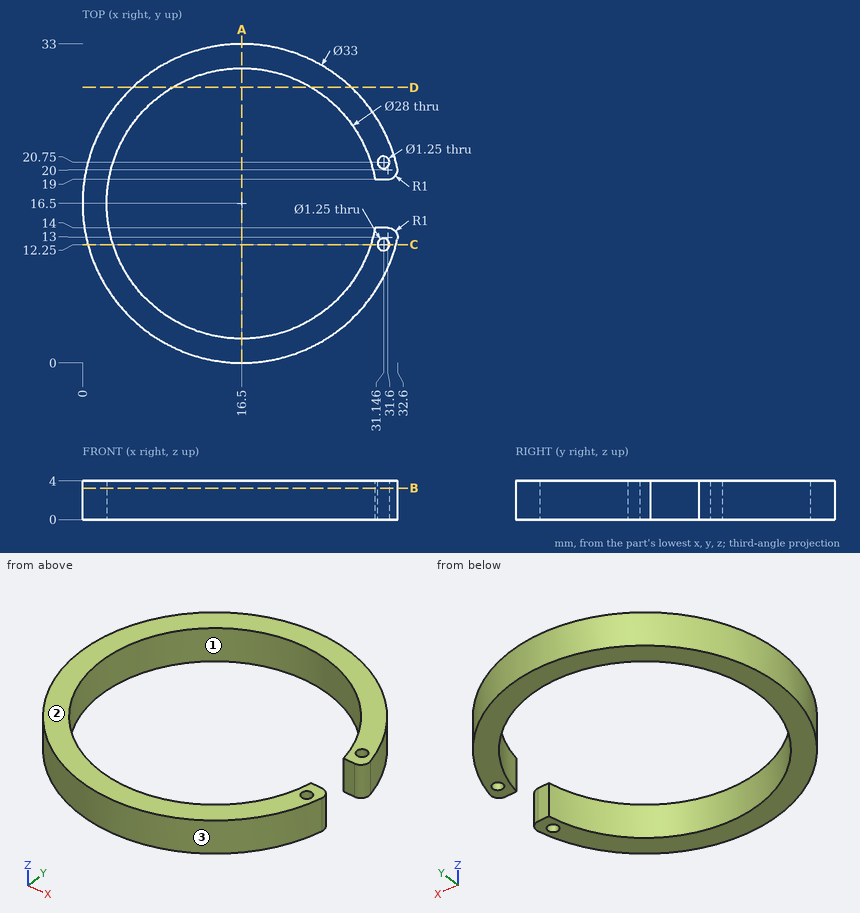
Print and shaded views of the part. All mm, measured from the part's lowest x, y and z. Coordinates: 2 decimals unless noted, no trailing zeros. Loops run counter-clockwise (first coordinate to the right, second up) from the corner with the lowest first, then second, coordinate; pieces in that order, holes last. Notation, with made-up numbers: (-33, -7) -> (-29, -7) arc R23 ccw to (-29, 27) -> close; hole circle Ø5 at (-11.5, -7.75). An arc over 180 degrees is marked (long way). Use a Markdown table: item, result. Add a question column.
Item 1: Probe probe 1 along X at (y, z) = (12.25, 2.8); probe 2 along X at (y, z) = (4.5, 3.5) (1 decimal); probe 3 along Y at (x, z) = (7, 2.35) (1 decimal). List the from-to ranges inside material, lowest first.
Item 2: Band-saw the part on D-D on y = 28.5. Write the cut outline in (x, z) (1 decimal).
Item 3: Flat gauge pins, fed straight in: P1, Ø0.8, axis at x = 31.15, y = 20.75, coming from the +Z side; P2, Ø1.1, axis at x = 31, z = 1.5, coming from the -Y side; P3, Ø0.7, axis at x = 31, z = 3, coming from the +Y side (1 decimal). Where does each tip first touch, or does it go through?
Item 4: Pull direction X, two halves, no side cores. Call the marked faces 1, 2 and 3: +X half, -X half, draft (parallel to the pull), parting line (faces both ways), or undercut.
Item 5: Band-saw the part on C-C on y = 12.25. Write the cut outline in (x, z).
Item 6: Band-saw the part on A-A on x = 16.5. Write the cut outline in (y, z).
Item 7: Band-saw the part on B-B on z = 3.25. Give the number of separate pieces and of enclosed holes in the cut face, plus the area to 3 significant figures.
Geometry says:
| question | item | result |
|---|---|---|
| 1 | probe 1 | 0.56 to 3.16, 29.84 to 30.52, 31.77 to 32.44 |
| 1 | probe 2 | 5.2 to 9.3, 23.7 to 27.8 |
| 1 | probe 3 | 3 to 6.2, 26.8 to 30 |
| 2 | outline | (5.2, 0) -> (9.3, 0) -> (9.3, 4) -> (5.2, 4) -> close; (23.7, 0) -> (27.8, 0) -> (27.8, 4) -> (23.7, 4) -> close |
| 3 | P1 | through |
| 3 | P2 | y = 7.69 |
| 3 | P3 | y = 25 |
| 4 | face 1 | undercut |
| 4 | face 2 | draft |
| 4 | face 3 | parting line |
| 5 | outline | (0.56, 0) -> (3.16, 0) -> (3.16, 4) -> (0.56, 4) -> close; (29.84, 0) -> (30.52, 0) -> (30.52, 4) -> (29.84, 4) -> close; (31.77, 0) -> (32.44, 0) -> (32.44, 4) -> (31.77, 4) -> close |
| 6 | outline | (0, 0) -> (2.5, 0) -> (2.5, 4) -> (0, 4) -> close; (30.5, 0) -> (33, 0) -> (33, 4) -> (30.5, 4) -> close |
| 7 | separate pieces | 1 |
| 7 | enclosed holes | 2 |
| 7 | area | 224 mm² |
